Could you check a few things on this model? Use its own coordinates, in mm. A direction names the side the tool comes from. Round coordinates to 2 decimals unless told otherwise and drop trailing zeros. Write each loop counter-clockwise with the first axis right and the second up, starting at its lowest first coordinate (ties: lowest second). Pieces come first, ordered by that corner, then holes. Notation, with made-up numbers: M 42,33 L 85,33 A28 ccw 85,65 Z; hole C 1,74 d8. An arc over 180 degrees is marked long. One line per item, written item: value. Start each with the question number.
(1) I'm going to push a flat-ended pin straight in: pin 1 Ø1 at (y, z) = (16.5, 4.5) entering from +X. Where does the tip first touch, or does it pass through?
(2) I want a section at B-B on z = -21.5. Please give me the cut outline in (x, y).
(3) Thinking about a two-plate mould opening in Z: for faces 4 (the face through (115.05, -33.58, -29.94)), 5 (the face through (115.668, 33.254, 25.301)), 6 (the face through (115.668, -33.254, -34.699)), which applies, released by +Z, released by -Z, zero draft, split by the parting line, or undercut?
(4) If I drill on L1, parallel to Z at x = 147, y = 16.5; L2, parallel to X at y = -28.5, z = -9.5; L3, parallel to Z at x = 147, y = -26, over which ranges is the centre line in solid material (lowest first)?
(5) Which directions (+Z, -Z, +X, -X, +Y, -Y) give clear straight access to the entire face, cutting with the end or side of a thin tool? Please do faces 1 (the face through (115.032, -33.279, -25.285)), 2 (the face through (88.267, 0, 0)), 3 (the face through (115.033, 33.295, -25.301)).
(6) I want a section at A-A on z = -28.5. Please give me the cut outline in (x, y).
```python
from build123d import *

# Parameters (mm, degrees)
BOSS_EXTRUDE1_DEPTH = 35
CUT_EXTRUDE1_DEPTH  = 70
CUT_EXTRUDE2_START  = -70
CUT_EXTRUDE2_DEPTH  = 70
FILLET3_R           = 1


# Read off the part's stored shape, not the designer's step: Cut-Extrude2
with BuildPart() as part:
    # Sketch2 → Boss-Extrude1 (new, symmetric)
    with BuildSketch(Plane(origin=(0, 0, 0), x_dir=(1, 0, 0), z_dir=(0, 1, 0))):
        Polygon((0, 0), (0, 70), (159.267236843, 70), (159.267236843, 60), (88.267236843, 60), (88.267236843, 10), (159.267236843, 10), (159.267236843, 0), align=None)
    extrude(amount=BOSS_EXTRUDE1_DEPTH, both=True)

    # Sketch3 → Cut-Extrude1 (cut)
    with BuildSketch(Plane.XY):
        Polygon((92.712686328, 35), (159.267236843, 30.767300383), (159.267236843, 35), align=None)
        Polygon((92.712686328, -35), (159.267236843, -30.767300383), (159.267236843, -35), align=None)
    extrude(amount=-CUT_EXTRUDE1_DEPTH, mode=Mode.SUBTRACT)

    # Cut-Extrude2 outline → Cut-Extrude2 (cut)
    with BuildSketch(Plane.XY.offset(CUT_EXTRUDE2_START)):
        with BuildLine():
            Line((159.267236843, 30.767300383), (138.20045286, 32.107094098))
            ThreePointArc((138.20045286, 32.107094098), (153.530375436, 19.200747894), (159.267236843, 0))
            Line((159.267236843, 0), (159.267236843, 30.767300383))
        make_face()
        with BuildLine():
            Line((159.267236843, -30.767300383), (159.267236843, 0))
            ThreePointArc((159.267236843, 0), (153.530375436, -19.200747894), (138.20045286, -32.107094098))
            Line((138.20045286, -32.107094098), (159.267236843, -30.767300383))
        make_face()
    extrude(amount=CUT_EXTRUDE2_DEPTH, mode=Mode.SUBTRACT)

    # Fillet3
    fillet3_edges = [part.edges().sort_by_distance(p)[0] for p in [
        (88.267236843, -35, -35),
        (46.356343164, -35, 0),
        (0, 0, 0),
        (0, 0, -70),
        (88.267236843, 0, -60),
        (88.267236843, 0, -10),
        (88.267236843, 35, -35),
        (90.489961586, 35, -60),
        (46.356343164, -35, -70),
        (90.489961586, -35, -10),
        (92.712686328, -35, -5),
        (90.489961586, 35, -10),
        (46.356343164, 35, -70),
        (92.712686328, 35, -5),
        (0, 35, -35),
        (92.712686328, 35, -65),
        (115.456569594, 33.553547049, -10),
        (115.456569594, 33.553547049, -70),
        (115.456569594, 33.553547049, 0),
        (92.712686328, -35, -65),
        (115.456569594, -33.553547049, -60),
        (46.356343164, 35, 0),
        (138.20045286, 32.107094098, -5),
        (115.456569594, 33.553547049, -60),
        (115.456569594, -33.553547049, 0),
        (115.456569594, -33.553547049, -10),
        (115.456569594, -33.553547049, -70),
        (153.530375436, -19.200747894, -60),
        (138.20045286, -32.107094098, -65),
        (153.530375436, 19.200747894, -70),
        (138.20045286, -32.107094098, -5),
        (153.530375436, 19.200747894, -10),
        (138.20045286, 32.107094098, -65),
        (153.530375436, 19.200747894, 0),
        (0, -35, -35),
        (90.489961586, -35, -60),
    ]]
    fillet(fillet3_edges, radius=FILLET3_R)


with BuildPart() as part_1:
    # Body-Move/Copy1: moved
    add(part.part.moved(Location((0, 0, 35))))


solid = part_1.part
```
Found:
1. pin 1: stops at x = 88.27
2. outline: M 0,-34 A1 ccw 1,-35 L 87.27,-35 A1 ccw 88.27,-34 L 88.27,34 A1 ccw 87.27,35 L 1,35 A1 ccw 0,34 Z
3. face 4: zero draft
3. face 5: undercut
3. face 6: released by -Z
4. L1: z = -35 to -25, 25 to 35
4. L2: x = 0 to 88.27
4. L3: z = -34.84 to -25.16, 25.16 to 34.84
5. face 1: +X, -Y
5. face 2: +X, +Y, -Y
5. face 3: +X, +Y
6. outline: M 0,-34 A1 ccw 1,-35 L 92.71,-35 L 138.02,-32.12 A1 ccw 138.36,-32.04 A35 ccw 138.36,32.04 A1 ccw 138.02,32.12 L 92.71,35 L 1,35 A1 ccw 0,34 Z
